from build123d import *

# Parameters (mm, degrees)
BOSS_EXTRUDE2_DEPTH = 1.5875
SKETCH2_W           = 10.414
SKETCH2_H           = 1.27
SKETCH2_W_2         = 5.9944
SKETCH2_H_2         = 1.016
SKETCH2_W_3         = 2.413
SKETCH2_H_3         = 1.3716
CUT_EXTRUDE1_DEPTH  = 57.702519048
SKETCH3_W           = 10.16
SKETCH3_H           = 0.635
SKETCH3_W_2         = 10.414
CUT_EXTRUDE2_DEPTH  = 57.702519048
SKETCH4_W           = 17.78
SKETCH4_H           = 0.254
CUT_EXTRUDE3_DEPTH  = 57.702519048
SKETCH5_W           = 10.414
SKETCH5_H           = 0.254
CUT_EXTRUDE4_DEPTH  = 57.602133313


with BuildPart() as part:
    # Sketch1 → Boss-Extrude2 (new, symmetric)
    with BuildSketch(Plane(origin=(0, 0, 0), x_dir=(1, 0, 0), z_dir=(0, 1, 0))):
        Polygon((-49.022, -7.3025), (-49.022, 0), (-49.022, 7.3025), (-51.943, 7.3025), (-51.943, 14.1605), (-41.529, 14.1605), (-41.529, 17.0815), (-31.369, 17.0815), (-31.369, 22.5171), (-13.589, 22.5171), (-13.589, 17.0815), (-3.429, 17.0815), (-3.429, 22.5171), (14.351, 22.5171), (14.351, 17.0815), (24.511, 17.0815), (24.511, 13.9065), (30.5054, 13.9065), (30.5054, 17.0815), (40.9194, 17.0815), (40.9194, 14.2621), (43.3324, 14.2621), (43.3324, 7.3025), (46.2534, 7.3025), (46.2534, 0), (46.2534, -7.3025), (43.3324, -7.3025), (43.3324, -14.1605), (35.8394, -14.1605), (35.8394, -19.5961), (4.0894, -19.5961), (4.0894, -14.1605), (-9.779, -14.1605), (-9.779, -19.5961), (-41.529, -19.5961), (-41.529, -14.1605), (-51.943, -14.1605), (-51.943, -7.3025), align=None)
    extrude(amount=BOSS_EXTRUDE2_DEPTH, both=True)

    # Sketch2 → Cut-Extrude1 (cut, through all)
    with BuildSketch(Plane(origin=(0, 1.5875, 0), x_dir=(1, 0, 0), z_dir=(0, 1, 0))):
        with Locations((-46.736, 13.5255)):
            Rectangle(SKETCH2_W, SKETCH2_H)
        with Locations((27.5082, 13.3985)):
            Rectangle(SKETCH2_W_2, SKETCH2_H_2)
        with Locations((42.1259, 13.5763)):
            Rectangle(SKETCH2_W_3, SKETCH2_H_3)
    extrude(amount=-CUT_EXTRUDE1_DEPTH, mode=Mode.SUBTRACT)

    # Sketch3 → Cut-Extrude2 (cut, through all)
    with BuildSketch(Plane(origin=(0, 1.5875, 0), x_dir=(1, 0, 0), z_dir=(0, 1, 0))):
        with Locations((-36.449, 16.764)):
            Rectangle(SKETCH3_W, SKETCH3_H)
        with Locations((-8.509, 16.764)):
            Rectangle(SKETCH3_W, SKETCH3_H)
        with Locations((19.431, 16.764)):
            Rectangle(SKETCH3_W, SKETCH3_H)
        with Locations((35.7124, 16.764)):
            Rectangle(SKETCH3_W_2, SKETCH3_H)
    extrude(amount=-CUT_EXTRUDE2_DEPTH, mode=Mode.SUBTRACT)

    # Sketch4 → Cut-Extrude3 (cut, through all)
    with BuildSketch(Plane(origin=(0, 1.5875, 0), x_dir=(1, 0, 0), z_dir=(0, 1, 0))):
        with Locations((-22.479, 22.3901)):
            Rectangle(SKETCH4_W, SKETCH4_H)
        with Locations((5.461, 22.3901)):
            Rectangle(SKETCH4_W, SKETCH4_H)
    extrude(amount=-CUT_EXTRUDE3_DEPTH, mode=Mode.SUBTRACT)

    # Sketch5 → Cut-Extrude4 (cut, through all)
    with BuildSketch(Plane(origin=(0, 1.5875, 0), x_dir=(1, 0, 0), z_dir=(0, 1, 0))):
        with Locations((35.7124, 16.3195)):
            Rectangle(SKETCH5_W, SKETCH5_H)
    extrude(amount=-CUT_EXTRUDE4_DEPTH, mode=Mode.SUBTRACT)


solid = part.part
Source: CAD feature listing. Evaluate the final solid. Frame: model axes, mm. A direction names the side the tool comes from. Give positions to 0.01 mm unless a question says otherwise; leave off trailing zeros. Write each loop counter-clockwise with the first axis right and the second up, starting at its lowest first coordinate (ties: lowest second). Pieces come first, ordered by that corner, then holes. Notation, with made-up numbers: M 6,-17 L 49,-17 A34 ccw 49,16 Z; hole C 75.5,4.5 d6. An arc over 180 degrees is marked long. Answer as a JSON object with one key per item and string values.
Q1. Contact query for flat-ended pins moving along their axis: P1, Ø1, axis at y = -0.5, z = 11, coming from the +X side; P2, Ø1, axis at x = -38.5, y = 0.5, coming from the -Z side; P3, Ø1.5, axis at x = -50, y = 0, coming from the +Z side. Output: stop coordinate, or through.
Geometry check:
{"P1": "stops at x = 43.33", "P2": "stops at z = -16.45", "P3": "stops at z = 14.16"}
Q2. Ray query, line 1 along X through (y, z) = (-1.4, -15); line 2 along X through (y, z) = (-0.85, 16.5); line 3 along Z through (x, y) = (29.5, 0.5). Return the intervals inside material, ascending.
Geometry check:
{"line 1": "x = -41.53 to 24.51, 30.51 to 40.92", "line 2": "x = -41.53 to -9.78, 4.09 to 35.84", "line 3": "z = -12.89 to 19.6"}
Q3. Mould query, pull axis Z, two halves, no side actions, for faces 1 (the face through (-51, 0, 7.302)), 2 (the face through (24.511, 0, -15)), 3 (the face through (27, 0, -12.89)). Classes: +Z half, -Z half, draft (parallel to the pull), parting line (faces both ways), or undercut.
Geometry check:
{"face 1": "undercut", "face 2": "draft", "face 3": "-Z half"}
Q4. Access query for faces 4 (the face through (35.839, 0, 17)), 5 (the face through (-31.369, 0, -19)), 6 (the face through (-50, 0, -7.302)), 7 (the face through (-13.589, 0, -19)). Directions: +Z, -Z, +X, -X, +Y, -Y. A direction counts if a zero-diameter tool reaches every point of the face in a straight line with its end or side. Return the directions, or none.
Geometry check:
{"face 4": "+Z, +X, +Y, -Y", "face 5": "-Z, -X, +Y, -Y", "face 6": "-X, +Y, -Y", "face 7": "-Z, +Y, -Y"}
Q5. Cut plane C-C, the plane z = 9. Return the cut outline in (x, y), then the cut area to 4 significant figures.
Geometry check:
{"outline": "M -51.94,-1.59 L 43.33,-1.59 L 43.33,1.59 L -51.94,1.59 Z", "area": "302.5 mm^2"}
Q6. Cut plane B-B, the plane z = -14. Return the cut outline in (x, y).
Geometry check:
{"outline": "M -41.53,-1.59 L 24.51,-1.59 L 24.51,1.59 L -41.53,1.59 Z; M 30.51,-1.59 L 40.92,-1.59 L 40.92,1.59 L 30.51,1.59 Z"}
Q7. Cut plane A-A, the plane z = 17. Return the cut outline in (x, y).
Geometry check:
{"outline": "M -41.53,-1.59 L -9.78,-1.59 L -9.78,1.59 L -41.53,1.59 Z; M 4.09,-1.59 L 35.84,-1.59 L 35.84,1.59 L 4.09,1.59 Z"}
